Model file for the job. Use its own axes, mm. A direction names the side the tool comes from. Give positions to 0.01 mm unless a question says otherwise; leave off trailing zeros. Order: outer loops, then holes, each group sorted by start corner. A loop starts at its lowest first (then second) coordinate and runs counter-clockwise, first axis right, second up. Notation, with made-up numbers: (46.25, 71.5) - (98.25, 71.5) arc R10 cw to (98.25, 78.5) - close; hole circle Ø3 at (29.5, 73.25). An arc over 180 degrees is marked (long way). Use CSV: the item, a comma, the result in double quotes. Start each with the question number.
(1) Tool access for faces 1 (the flat face through (-25, -32, 0)), 2 (the flat face through (0.1, 5, -4.3)): list every direction of +Z, -Z, +X, -X, +Y, -Y with a clear straight run to the whole face (end or side of a thin tool).
(2) Band-saw the part on A-A, the plane z = 0. Give the cut face in (x, y), then the cut area to 3 significant figures.
(3) Band-saw the part on C-C, the plane z = -6. Give the cut face in (x, y).
(4) Probe L1, parallel to Y at x = 10, z = -15; L2, parallel to Y at x = -5, z = 5.5; L3, parallel to X at y = 3.5, z = -3.5. List the from-to ranges inside material, lowest first.
(5) Band-saw the part on D-D, the plane x = -14. Give the cut face in (y, z), then the cut area to 3 significant figures.
(6) Band-saw the part on B-B, the plane x = 0. Give the cut face in (y, z), then the cut area to 3 significant figures.
from build123d import *

# Parameters (mm, degrees)
F0_W     = 50
F0_H     = 50
F1_DEPTH = 65
F2_R     = 10
F3_DEPTH = 5
F4_R     = 4
F5_DEPTH = 20
F6_SIZE  = 3


with BuildPart() as f1:
    # F0 (on Front) → F1 (new body)
    with BuildSketch(Plane.XZ):
        Rectangle(F0_W, F0_H)
    extrude(amount=F1_DEPTH)

    # F2 (on face) → F3 (join)
    with BuildSketch(Plane(origin=(0, 0, 0), x_dir=(-1, 0, 0), z_dir=(0, 1, 0))):
        Circle(F2_R)
    extrude(amount=F3_DEPTH)

    # F4 (on face) → F5 (join)
    with BuildSketch(Plane(origin=(0, 5, 0), x_dir=(-1, 0, 0), z_dir=(0, 1, 0))):
        Circle(F4_R)
    extrude(amount=F5_DEPTH)

    # F6
    f6_edges = [f1.edges().sort_by_distance(p)[0] for p in [
        (-25, -32.5, 25),
        (-25, -32.5, -25),
        (25, -32.5, -25),
        (25, -32.5, 25),
    ]]
    chamfer(f6_edges, length=F6_SIZE)


solid = f1.part
Answer block:
1,face 1,"+Z, -Z, -X, +Y, -Y"
1,face 2,"+Y"
2,outline,"(-25, -65) - (25, -65) - (25, 0) - (10, 0) - (10, 5) - (4, 5) - (4, 25) - (-4, 25) - (-4, 5) - (-10, 5) - (-10, 0) - (-25, 0) - close"
2,area,"3,510 mm2"
3,outline,"(-25, -65) - (25, -65) - (25, 0) - (8, 0) - (8, 5) - (-8, 5) - (-8, 0) - (-25, 0) - close"
4,L1,"y = -65 to 0"
4,L2,"y = -65 to 5"
4,L3,"x = -9.37 to 9.37"
5,outline,"(-65, -25) - (0, -25) - (0, 25) - (-65, 25) - close"
5,area,"3,250 mm2"
6,outline,"(-65, -25) - (0, -25) - (0, -10) - (5, -10) - (5, -4) - (25, -4) - (25, 4) - (5, 4) - (5, 10) - (0, 10) - (0, 25) - (-65, 25) - close"
6,area,"3,510 mm2"
